For this review, take the finished solid that the model builds, in its own axes (mm). A direction names the side the tool comes from. Give positions to 0.01 mm unless a question says otherwise; leave off trailing zeros. Order: outer loops, then holes, each group sorted by start corner. A loop starts at its lowest first (then second) coordinate and runs counter-clockwise, first axis right, second up. Notation, with made-up numbers: (59, -22.75) - (111, -22.75) arc R19 cw to (111, -17.75) - close; hole circle Ø5 at (17.5, 49.25). An arc over 180 degrees is marked (long way). Use a Markdown table: item, result. Add a question column.
1) Clearance check with a flat-ended pin moving along its axis: P1, Ø1.5, axis at x = 80.5, z = 2, coming from the -Y side. State where the tip first meets the part, or that it passes through.
2) Machinability: for faces 1 (the face through (301.8, 13.54, 1.48)), 2 (the face through (193, 97, 0)), which of the approach directions +Z, -Z, +X, -X, +Y, -Y give a long, thin tool a straight path to every point of the face, cutting with its end or side? Answer none if there is none.
3) We need section B-B on y = 150. Write out the cut boundary in (x, z), then the cut area to 3 significant figures.
4) We need section D-D on z = 0.9. Give the number of separate pieces and of enclosed holes in the cut face, then the cut area to 3 significant figures.
5) We need section A-A on x = 345. Write out the cut boundary in (y, z).
6) Wall thickness on L1, parallel to X at y = 88, z = 0.5; L2, parallel to Y at x = 370.92, z = 0.75; L3, parallel to Y at x = 40.5, z = 2.85: over which ranges is each line inside the solid? List them lowest first.
7) We need section C-C on x = 116. Write out the cut boundary in (y, z).
8) Mouldability with a two-part tool opening along X and no side actions: class faces 3 (the face through (193, 97, 3)), 4 (the face through (150.236, 31.765, 1.479)), 5 (the face through (79.87, 13.93, 1.48)) as released by +X, released by -X, zero draft, split by the parting line, or undercut.
```python
from build123d import *

# Parameters (mm, degrees)
SKETCH1_R           = 1.5
SKETCH1_R_2         = 6
SKETCH1_W           = 30
SKETCH1_H           = 3
SKETCH1_W_2         = 3
SKETCH1_H_2         = 30
BOSS_EXTRUDE1_DEPTH = 3


with BuildPart() as part:
    # Sketch1 → Boss-Extrude1 (new body)
    with BuildSketch(Plane(origin=(-12.611770594, -16.696126479, 0), x_dir=(0, -1, 0), z_dir=(0, 0, 1))):
        Polygon((-213.696126479, 12.611770594), (-213.696126479, 393.451770594), (-16.696126479, 393.451770594), (-16.696126479, 343.451770594), (-44.166313492, 284.541764437), (-52.636925092, 203.031770594), (-44.166313492, 121.521776752), (-16.696126479, 62.611770594), (-16.696126479, 12.611770594), align=None)
        with Locations((-200.179850585, 21.811770594)):
            Circle(SKETCH1_R, mode=Mode.SUBTRACT)
        with Locations((-58.093278212, 312.31748488)):
            Circle(SKETCH1_R, mode=Mode.SUBTRACT)
        with Locations((-200.196126479, 383.531770594)):
            Circle(SKETCH1_R, mode=Mode.SUBTRACT)
        with Locations((-71.696126479, 383.531770594)):
            Circle(SKETCH1_R, mode=Mode.SUBTRACT)
        with Locations((-58.136861316, 93.744627737)):
            Circle(SKETCH1_R, mode=Mode.SUBTRACT)
        with Locations((-71.679850585, 21.811770594)):
            Circle(SKETCH1_R, mode=Mode.SUBTRACT)
        with Locations((-77.241301287, 202.611770594)):
            Circle(SKETCH1_R_2, mode=Mode.SUBTRACT)
        with Locations((-171.679850585, 21.811770594)):
            Rectangle(SKETCH1_W, SKETCH1_H, mode=Mode.SUBTRACT)
        with Locations((-101.679850585, 21.811770594)):
            Rectangle(SKETCH1_W, SKETCH1_H, mode=Mode.SUBTRACT)
        with Locations((-58.093278212, 57.316056309)):
            Rectangle(SKETCH1_W_2, SKETCH1_H_2, mode=Mode.SUBTRACT)
        with Locations((-58.136861316, 130.173199166)):
            Rectangle(SKETCH1_W_2, SKETCH1_H_2, mode=Mode.SUBTRACT)
        with Locations((-58.136925092, 203.030342023)):
            Rectangle(SKETCH1_W_2, SKETCH1_H_2, mode=Mode.SUBTRACT)
        with Locations((-58.093278212, 275.88748488)):
            Rectangle(SKETCH1_W_2, SKETCH1_H_2, mode=Mode.SUBTRACT)
        with Locations((-58.093278212, 348.74748488)):
            Rectangle(SKETCH1_W_2, SKETCH1_H_2, mode=Mode.SUBTRACT)
        with Locations((-101.696126479, 383.531770594)):
            Rectangle(SKETCH1_W, SKETCH1_H, mode=Mode.SUBTRACT)
        with Locations((-171.696126479, 383.531770594)):
            Rectangle(SKETCH1_W, SKETCH1_H, mode=Mode.SUBTRACT)
    extrude(amount=BOSS_EXTRUDE1_DEPTH)


solid = part.part
```
Checked values:
| question | item | result |
|---|---|---|
| 1 | P1 | y = 13.87 |
| 2 | face 1 | +Z, -Z, -Y |
| 2 | face 2 | -Z, +X, -X, +Y, -Y |
| 3 | outline | (0, 0) - (7.7, 0) - (7.7, 3) - (0, 3) - close; (10.7, 0) - (369.42, 0) - (369.42, 3) - (10.7, 3) - close; (372.42, 0) - (380.84, 0) - (380.84, 3) - (372.42, 3) - close |
| 3 | area | 1,120 mm² |
| 4 | separate pieces | 1 |
| 4 | enclosed holes | 16 |
| 4 | area | 67,300 mm² |
| 5 | outline | (0, 0) - (39.9, 0) - (39.9, 3) - (0, 3) - close; (42.9, 0) - (197, 0) - (197, 3) - (42.9, 3) - close |
| 6 | L1 | 0 to 7.7, 10.7 to 369.42, 372.42 to 380.84 |
| 6 | L2 | 0 to 53.5, 56.5 to 70, 100 to 140, 170 to 182, 185 to 197 |
| 6 | L3 | 0 to 39.9, 42.9 to 197 |
| 7 | outline | (28.21, 0) - (39.94, 0) - (39.94, 3) - (28.21, 3) - close; (42.94, 0) - (197, 0) - (197, 3) - (42.94, 3) - close |
| 8 | face 3 | zero draft |
| 8 | face 4 | undercut |
| 8 | face 5 | undercut |
